Source: CAD feature listing. Evaluate the final solid. Frame: model axes, mm. Face numbers are marked on the shaded views. A direction names the side the tool comes from. Round coordinates to 2 decimals unless told otherwise and drop trailing zeros. Write each loop counter-clockwise with the first axis right and the second up, starting at its lowest first coordinate (ties: lowest second). Pieces come first, ordered by that corner, then holes. Notation, with made-up numbers: M 37.5,-9 L 61.5,-9 A15 ccw 61.5,5 Z; hole C 56,-11.75 d10. An arc over 180 degrees is marked long. Answer in a Markdown table with one row per item. Add a question column.
Item 1: Mould query, pull axis Z, two halves, no side actions, for the marked faces 4, 5 and 6. Classes: released by +Z, released by -Z, zero draft, split by the parting line, or undercut.
Item 2: Cut plane C-C on x = 22. Return loops of the section in (y, z), and give its area (3 significant figures).
Item 3: Cut plane D-D on y = 3. Return loops of the section in (x, z), and give its area (3 significant figures).
Item 4: Material intervals for probe 1 along Z at (x, y) = (36, -3.25); probe 2 along Y at (x, z) = (5.5, -7.75); probe 3 along Y at (x, z) = (39.5, -7), sorted ascending.
Item 5: Cut plane A-A on y = -1.5. Return loops of the section in (x, z), and give its area (3 significant figures).
Item 6: Set-up query: the marked faces 1, 2 and 3. Return all of +Z, -Z, +X, -X, +Y, -Y with unobstructed straight access to the full face (end or side cutting, diameter ignored); none if empty.
Item 7: Contact query for flat-ended pins moving along their axis: pin 1 (1 mm diameter, centred on x = 12, z = -2, fed in from +Y); pin 2 (1.7 mm diameter, centred on y = -2, z = -14, fed in from -X); pin 3 (0.7 mm diameter, centred on x = 16, y = -5.5, fed in from -Z); pin 4 (2 mm diameter, centred on x = 27.5, y = 3.5, fed in from -Z). Output: stop coordinate, or through.
Item 8: Cut plane B-B on z = -7.75. Return loops of the section in (x, y).
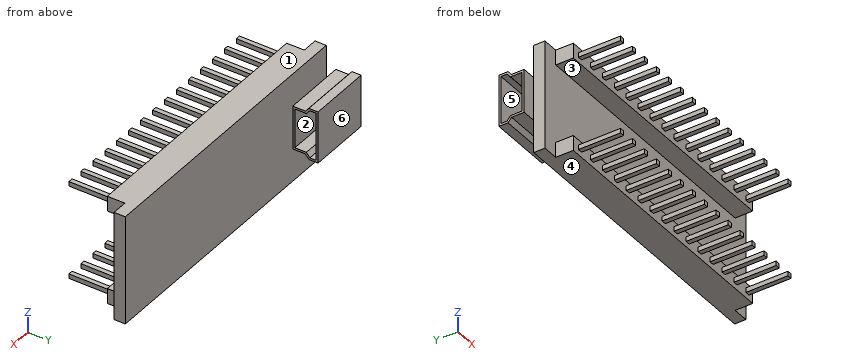
from build123d import *

# Parameters (mm, degrees)
SKETCH1_W                = 42
SKETCH1_H                = 15.5
BOSS_EXTRUDE1_DEPTH      = 1.6
EXTRUDE_THIN1_START      = -7
EXTRUDE_THIN1_DEPTH      = 9
SKETCH3_W                = 18.75
SKETCH3_H                = 2.148280867
BOSS_EXTRUDE2_DEPTH      = 2.5
SKETCH4_W                = 0.654719532
SKETCH4_H                = 0.654719531
BOSS_EXTRUDE3_DEPTH      = 6
LPATTERN1_COUNT          = 15
LPATTERN1_PITCH          = 2.5
MIRROR4_COPY_1_SKETCH_W  = 0.654719532
MIRROR4_COPY_1_SKETCH_H  = 0.654719531
MIRROR4_COPY_1_DEPTH     = 6
MIRROR4_COPY_2_SKETCH_W  = 0.654719532
MIRROR4_COPY_2_SKETCH_H  = 0.654719531
MIRROR4_COPY_2_DEPTH     = 6
MIRROR4_COPY_3_SKETCH_W  = 0.654719532
MIRROR4_COPY_3_SKETCH_H  = 0.654719531
MIRROR4_COPY_3_DEPTH     = 6
MIRROR4_COPY_4_SKETCH_W  = 0.654719532
MIRROR4_COPY_4_SKETCH_H  = 0.654719531
MIRROR4_COPY_4_DEPTH     = 6
MIRROR4_COPY_5_SKETCH_W  = 0.654719532
MIRROR4_COPY_5_SKETCH_H  = 0.654719531
MIRROR4_COPY_5_DEPTH     = 6
MIRROR4_COPY_6_SKETCH_W  = 0.654719532
MIRROR4_COPY_6_SKETCH_H  = 0.654719531
MIRROR4_COPY_6_DEPTH     = 6
MIRROR4_COPY_7_SKETCH_W  = 0.654719532
MIRROR4_COPY_7_SKETCH_H  = 0.654719531
MIRROR4_COPY_7_DEPTH     = 6
MIRROR4_COPY_8_SKETCH_W  = 0.654719532
MIRROR4_COPY_8_SKETCH_H  = 0.654719531
MIRROR4_COPY_8_DEPTH     = 6
MIRROR4_COPY_9_SKETCH_W  = 0.654719532
MIRROR4_COPY_9_SKETCH_H  = 0.654719531
MIRROR4_COPY_9_DEPTH     = 6
MIRROR4_COPY_10_SKETCH_W = 0.654719532
MIRROR4_COPY_10_SKETCH_H = 0.654719531
MIRROR4_COPY_10_DEPTH    = 6
MIRROR4_COPY_11_SKETCH_W = 0.654719532
MIRROR4_COPY_11_SKETCH_H = 0.654719531
MIRROR4_COPY_11_DEPTH    = 6
MIRROR4_COPY_12_SKETCH_W = 0.654719532
MIRROR4_COPY_12_SKETCH_H = 0.654719531
MIRROR4_COPY_12_DEPTH    = 6
MIRROR4_COPY_13_SKETCH_W = 0.654719532
MIRROR4_COPY_13_SKETCH_H = 0.654719531
MIRROR4_COPY_13_DEPTH    = 6
MIRROR4_COPY_14_SKETCH_W = 0.654719532
MIRROR4_COPY_14_SKETCH_H = 0.654719531
MIRROR4_COPY_14_DEPTH    = 6


with BuildPart() as part:
    # Sketch1 → Boss-Extrude1 (new body)
    with BuildSketch(Plane(origin=(0, 0, 0), x_dir=(1, 0, 0), z_dir=(0, 1, 0))):
        with Locations((21, 7.75)):
            Rectangle(SKETCH1_W, SKETCH1_H)
    extrude(amount=BOSS_EXTRUDE1_DEPTH)

    # Sketch2 → Extrude-Thin1 (add)
    with BuildSketch(Plane.ZY.offset(EXTRUDE_THIN1_START)):
        Polygon((-7.75, 1.6), (-10.85, 1.6), (-10.85, 3.4), (-11.45, 3.9), (-11.45, 5.2), (-7.75, 5.2), (-7.75, 4.9), (-11.15, 4.9), (-11.15, 4.040512484), (-10.55, 3.540512484), (-10.55, 1.9), (-7.75, 1.9), align=None)
    extrude_thin1 = extrude(amount=EXTRUDE_THIN1_DEPTH)

    # Mirror1: Extrude-Thin1 across plane
    add(extrude_thin1.mirror(Plane.XY.offset(-7.75)))

    # Sketch3 → Boss-Extrude2 (add)
    with BuildSketch(Plane.XZ):
        with Locations((11.625, -1.074140433)):
            Rectangle(SKETCH3_W, SKETCH3_H)
        with Locations((30.375, -1.074140433)):
            Rectangle(SKETCH3_W, SKETCH3_H)
    boss_extrude2 = extrude(amount=BOSS_EXTRUDE2_DEPTH)

    # Sketch4 → Boss-Extrude3 (add)
    with BuildSketch(Plane.XZ.offset(2.5)):
        with Locations((3.64534799, -1.074140433)):
            Rectangle(SKETCH4_W, SKETCH4_H)
    boss_extrude3 = extrude(amount=BOSS_EXTRUDE3_DEPTH)

    # LPattern1: Boss-Extrude3 ×15
    with Locations(*[(i * LPATTERN1_PITCH, 0, 0) for i in range(1, LPATTERN1_COUNT)]):
        add(boss_extrude3)

    # Mirror3: Boss-Extrude2 across plane
    add(boss_extrude2.mirror(Plane.XY.offset(-7.75)))

    # Mirror4: Boss-Extrude3 across plane
    add(boss_extrude3.mirror(Plane.XY.offset(-7.75)))

    # Mirror4 copy 1 sketch → Mirror4 copy 1 (add)
    with BuildSketch(Plane(origin=(2.5, -2.5, -15.5), x_dir=(1, 0, 0), z_dir=(0, -1, 0))):
        with Locations((3.64534799, 1.074140433)):
            Rectangle(MIRROR4_COPY_1_SKETCH_W, MIRROR4_COPY_1_SKETCH_H)
    extrude(amount=MIRROR4_COPY_1_DEPTH)

    # Mirror4 copy 2 sketch → Mirror4 copy 2 (add)
    with BuildSketch(Plane(origin=(5, -2.5, -15.5), x_dir=(1, 0, 0), z_dir=(0, -1, 0))):
        with Locations((3.64534799, 1.074140433)):
            Rectangle(MIRROR4_COPY_2_SKETCH_W, MIRROR4_COPY_2_SKETCH_H)
    extrude(amount=MIRROR4_COPY_2_DEPTH)

    # Mirror4 copy 3 sketch → Mirror4 copy 3 (add)
    with BuildSketch(Plane(origin=(7.5, -2.5, -15.5), x_dir=(1, 0, 0), z_dir=(0, -1, 0))):
        with Locations((3.64534799, 1.074140433)):
            Rectangle(MIRROR4_COPY_3_SKETCH_W, MIRROR4_COPY_3_SKETCH_H)
    extrude(amount=MIRROR4_COPY_3_DEPTH)

    # Mirror4 copy 4 sketch → Mirror4 copy 4 (add)
    with BuildSketch(Plane(origin=(10, -2.5, -15.5), x_dir=(1, 0, 0), z_dir=(0, -1, 0))):
        with Locations((3.64534799, 1.074140433)):
            Rectangle(MIRROR4_COPY_4_SKETCH_W, MIRROR4_COPY_4_SKETCH_H)
    extrude(amount=MIRROR4_COPY_4_DEPTH)

    # Mirror4 copy 5 sketch → Mirror4 copy 5 (add)
    with BuildSketch(Plane(origin=(12.5, -2.5, -15.5), x_dir=(1, 0, 0), z_dir=(0, -1, 0))):
        with Locations((3.64534799, 1.074140433)):
            Rectangle(MIRROR4_COPY_5_SKETCH_W, MIRROR4_COPY_5_SKETCH_H)
    extrude(amount=MIRROR4_COPY_5_DEPTH)

    # Mirror4 copy 6 sketch → Mirror4 copy 6 (add)
    with BuildSketch(Plane(origin=(15, -2.5, -15.5), x_dir=(1, 0, 0), z_dir=(0, -1, 0))):
        with Locations((3.64534799, 1.074140433)):
            Rectangle(MIRROR4_COPY_6_SKETCH_W, MIRROR4_COPY_6_SKETCH_H)
    extrude(amount=MIRROR4_COPY_6_DEPTH)

    # Mirror4 copy 7 sketch → Mirror4 copy 7 (add)
    with BuildSketch(Plane(origin=(17.5, -2.5, -15.5), x_dir=(1, 0, 0), z_dir=(0, -1, 0))):
        with Locations((3.64534799, 1.074140433)):
            Rectangle(MIRROR4_COPY_7_SKETCH_W, MIRROR4_COPY_7_SKETCH_H)
    extrude(amount=MIRROR4_COPY_7_DEPTH)

    # Mirror4 copy 8 sketch → Mirror4 copy 8 (add)
    with BuildSketch(Plane(origin=(20, -2.5, -15.5), x_dir=(1, 0, 0), z_dir=(0, -1, 0))):
        with Locations((3.64534799, 1.074140433)):
            Rectangle(MIRROR4_COPY_8_SKETCH_W, MIRROR4_COPY_8_SKETCH_H)
    extrude(amount=MIRROR4_COPY_8_DEPTH)

    # Mirror4 copy 9 sketch → Mirror4 copy 9 (add)
    with BuildSketch(Plane(origin=(22.5, -2.5, -15.5), x_dir=(1, 0, 0), z_dir=(0, -1, 0))):
        with Locations((3.64534799, 1.074140433)):
            Rectangle(MIRROR4_COPY_9_SKETCH_W, MIRROR4_COPY_9_SKETCH_H)
    extrude(amount=MIRROR4_COPY_9_DEPTH)

    # Mirror4 copy 10 sketch → Mirror4 copy 10 (add)
    with BuildSketch(Plane(origin=(25, -2.5, -15.5), x_dir=(1, 0, 0), z_dir=(0, -1, 0))):
        with Locations((3.64534799, 1.074140433)):
            Rectangle(MIRROR4_COPY_10_SKETCH_W, MIRROR4_COPY_10_SKETCH_H)
    extrude(amount=MIRROR4_COPY_10_DEPTH)

    # Mirror4 copy 11 sketch → Mirror4 copy 11 (add)
    with BuildSketch(Plane(origin=(27.5, -2.5, -15.5), x_dir=(1, 0, 0), z_dir=(0, -1, 0))):
        with Locations((3.64534799, 1.074140433)):
            Rectangle(MIRROR4_COPY_11_SKETCH_W, MIRROR4_COPY_11_SKETCH_H)
    extrude(amount=MIRROR4_COPY_11_DEPTH)

    # Mirror4 copy 12 sketch → Mirror4 copy 12 (add)
    with BuildSketch(Plane(origin=(30, -2.5, -15.5), x_dir=(1, 0, 0), z_dir=(0, -1, 0))):
        with Locations((3.64534799, 1.074140433)):
            Rectangle(MIRROR4_COPY_12_SKETCH_W, MIRROR4_COPY_12_SKETCH_H)
    extrude(amount=MIRROR4_COPY_12_DEPTH)

    # Mirror4 copy 13 sketch → Mirror4 copy 13 (add)
    with BuildSketch(Plane(origin=(32.5, -2.5, -15.5), x_dir=(1, 0, 0), z_dir=(0, -1, 0))):
        with Locations((3.64534799, 1.074140433)):
            Rectangle(MIRROR4_COPY_13_SKETCH_W, MIRROR4_COPY_13_SKETCH_H)
    extrude(amount=MIRROR4_COPY_13_DEPTH)

    # Mirror4 copy 14 sketch → Mirror4 copy 14 (add)
    with BuildSketch(Plane(origin=(35, -2.5, -15.5), x_dir=(1, 0, 0), z_dir=(0, -1, 0))):
        with Locations((3.64534799, 1.074140433)):
            Rectangle(MIRROR4_COPY_14_SKETCH_W, MIRROR4_COPY_14_SKETCH_H)
    extrude(amount=MIRROR4_COPY_14_DEPTH)


solid = part.part
Results below:
| question | item | result |
|---|---|---|
| 1 | face 4 | released by -Z |
| 1 | face 5 | undercut |
| 1 | face 6 | zero draft |
| 2 | outline | M -2.5,-15.5 L 1.6,-15.5 L 1.6,0 L -2.5,0 L -2.5,-2.15 L 0,-2.15 L 0,-13.35 L -2.5,-13.35 Z |
| 2 | area | 35.5 mm2 |
| 3 | outline | M -2,-10.85 L 7,-10.85 L 7,-10.55 L -2,-10.55 Z; M -2,-4.95 L 7,-4.95 L 7,-4.65 L -2,-4.65 Z |
| 3 | area | 5.40 mm2 |
| 4 | probe 1 | -14.75 to -14.1, -1.4 to -0.75 |
| 4 | probe 2 | 0 to 1.9, 4.9 to 5.2 |
| 4 | probe 3 | 0 to 1.6 |
| 5 | outline | M 2.25,-15.5 L 39.75,-15.5 L 39.75,-13.35 L 2.25,-13.35 Z; M 2.25,-2.15 L 39.75,-2.15 L 39.75,0 L 2.25,0 Z |
| 5 | area | 161 mm2 |
| 6 | face 1 | +Z, +X, -X, +Y, -Y |
| 6 | face 2 | +X, -X |
| 6 | face 3 | +X, -X, -Y |
| 7 | pin 1 | y = 1.6 |
| 7 | pin 2 | x = 2.25 |
| 7 | pin 3 | z = -14.75 |
| 7 | pin 4 | through |
| 8 | outline | M -2,1.6 L 0,1.6 L 0,0 L 42,0 L 42,1.6 L 7,1.6 L 7,1.9 L -2,1.9 Z; M -2,4.9 L 7,4.9 L 7,5.2 L -2,5.2 Z |
